from build123d import *

# Parameters (mm, degrees)
SKETCH_1_W          = 4
SKETCH_1_H          = 6
EXTRUDE_1_DEPTH     = 8
EXTRUDE_START       = 8
SKETCH_1_3_W        = 4
SKETCH_1_3_H        = 6
EXTRUDE_2_DEPTH     = 30
CUT_EXTRUDE_1_DEPTH = 6


with BuildPart() as part:
    # Эскиз1 → Бобышка-Вытянуть1 (new body)
    with BuildSketch(Plane.XY):
        Polygon((0, 30), (0, 0), (15, 0), (15, 6), (8, 6), (8, 30), align=None)
        with Locations((4, 23)):
            Rectangle(SKETCH_1_W, SKETCH_1_H, mode=Mode.SUBTRACT)
        with Locations((4, 13)):
            Rectangle(SKETCH_1_W, SKETCH_1_H, mode=Mode.SUBTRACT)
    extrude(amount=EXTRUDE_1_DEPTH)

    # Эскиз1<3> → Бобышка-Вытянуть2 (add)
    with BuildSketch(Plane.XY.offset(EXTRUDE_START)):
        Polygon((8, 30), (4, 30), (4, 26), (6, 26), (6, 20), (4, 20), (4, 16), (6, 16), (6, 10), (4, 10), (4, 6), (8, 6), align=None)
        Polygon((4, 30), (0, 30), (0, 6), (4, 6), (4, 10), (2, 10), (2, 16), (4, 16), (4, 20), (2, 20), (2, 26), (4, 26), align=None)
        with Locations((2, 3)):
            Rectangle(SKETCH_1_3_W, SKETCH_1_3_H)
        with Locations((6, 3)):
            Rectangle(SKETCH_1_3_W, SKETCH_1_3_H)
    extrude(amount=EXTRUDE_2_DEPTH)

    # Эскиз2 → Вырез-Вытянуть1 (cut)
    with BuildSketch(Plane.XZ):
        with BuildLine():
            Line((4, 2), (12, 2))
            ThreePointArc((12, 2), (14, 4), (12, 6))
            Line((12, 6), (4, 6))
            ThreePointArc((4, 6), (2, 4), (4, 2))
        make_face()
    extrude(amount=-CUT_EXTRUDE_1_DEPTH, mode=Mode.SUBTRACT)


solid = part.part
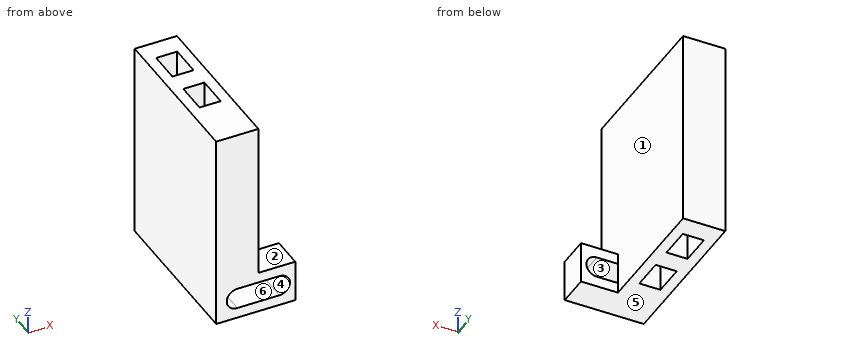
CAD build for the part. Positions are in the model's coordinates, mm. Face numbers are marked on the shaded views. A direction names the side the tool comes from. Round coordinates to 2 decimals unless told otherwise and drop trailing zeros. Loops run counter-clockwise (first coordinate to the right, second up) from the corner with the lowest first, then second, coordinate; pieces in that order, holes last.
(1) Two-plate mould, pull along Z, no slides. Class the marked faces 1, 2 and 3: +Z half, -Z half, draft (parallel to the pull), parting line (faces both ways), or undercut.
(2) Drop flat-ended pins along their axis: pin 1 (5 mm diameter, centred on y = 23.5, z = 17, fed in from +X); pin 2 (2 mm diameter, centred on x = 13, z = 5, fed in from +Y); pin 3 (6.5 mm diameter, centred on x = 12.5, y = 3.5, fed in from +Z). Give the stop position or say it passes through.
(3) Wall check: line 1 along Y through (x, z) = (3.5, 15.5); line 2 along Y through (x, z) = (5.5, 2.5); line 3 along X through (y, z) = (11, 18). Give the ranges that are in metal, low to high.
(4) Cut at B-B (x = 4.75). Give the cut face in (y, z), plus the area to 3 significant figures.
(5) Cut at D-D (x = 10.25). Give the cut face in (y, z).
(6) Which spindle directions (+Z, -Z, +X, -X, +Y, -Y) get a long thin tool onto all of the face, cutting with end or side? Do the marked faces 4, 5 and 6. Say none if no direction does.
(7) Cut at A-A (z = 4). Give the cut face in (x, y), plus the area to 3 significant figures.
(8) Cut at C-C (y = 25). Give the cut face in (x, z).
Findings below:
1. face 1: draft
1. face 2: +Z half
1. face 3: undercut
2. pin 1: stops at x = 8
2. pin 2: stops at y = 6
2. pin 3: stops at z = 8
3. line 1: y = 0 to 10, 16 to 20, 26 to 30
3. line 2: y = 6 to 10, 16 to 20, 26 to 30
3. line 3: x = 0 to 2, 6 to 8
4. outline: (0, 0) - (10, 0) - (10, 38) - (0, 38) - (0, 6) - (6, 6) - (6, 2) - (0, 2) - close; (16, 0) - (20, 0) - (20, 38) - (16, 38) - close; (26, 0) - (30, 0) - (30, 38) - (26, 38) - close
4. area: 660 mm2
5. outline: (0, 0) - (6, 0) - (6, 2) - (0, 2) - close; (0, 6) - (6, 6) - (6, 8) - (0, 8) - close
6. face 4: +Y, -Y
6. face 5: -Z, +X, -X, +Y, -Y
6. face 6: -Y
7. outline: (0, 0) - (2, 0) - (2, 6) - (8, 6) - (8, 30) - (0, 30) - close; (14, 0) - (15, 0) - (15, 6) - (14, 6) - close; hole (2, 10) - (6, 10) - (6, 16) - (2, 16) - close; hole (2, 20) - (6, 20) - (6, 26) - (2, 26) - close
7. area: 162 mm2
8. outline: (0, 0) - (2, 0) - (2, 38) - (0, 38) - close; (6, 0) - (8, 0) - (8, 38) - (6, 38) - close
